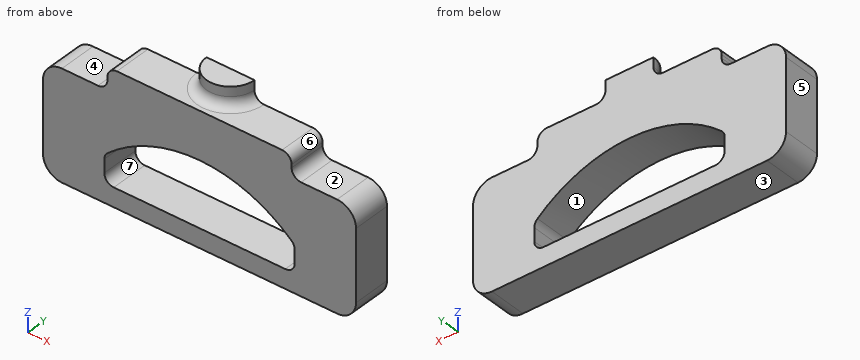
```python
from build123d import *

# Parameters (mm, degrees)
EXTRUDE1_DEPTH = 12.7
EXTRUDE2_DEPTH = 6.35
FILLET1_R      = 3.175


with BuildPart() as part:
    # Sketch1 → Extrude1 (new body)
    with BuildSketch(Plane(origin=(0, 0, 0), x_dir=(1, 0, 0), z_dir=(0, 1, 0))):
        with BuildLine():
            Line((0, 30.076477833), (0, 6.35))
            ThreePointArc((0, 6.35), (1.859871939, 1.859871939), (6.35, 0))
            Line((6.35, 0), (18.40185504, 0))
            ThreePointArc((18.40185504, 0), (20.64691907, -0.92993597), (21.57685504, -3.175))
            Line((21.57685504, -3.175), (21.57685504, -4.269827586))
            ThreePointArc((21.57685504, -4.269827586), (22.506791009, -6.514891616), (24.75185504, -7.444827586))
            Line((24.75185504, -7.444827586), (80.087569325, -7.444827586))
            ThreePointArc((80.087569325, -7.444827586), (82.332633356, -6.514891616), (83.262569325, -4.269827586))
            Line((83.262569325, -4.269827586), (83.262569325, -3.175))
            ThreePointArc((83.262569325, -3.175), (84.192505295, -0.92993597), (86.437569325, 0))
            Line((86.437569325, 0), (98.489424365, 0))
            ThreePointArc((98.489424365, 0), (102.979552425, 1.859871939), (104.839424365, 6.35))
            Line((104.839424365, 6.35), (104.839424365, 30.076477833))
            ThreePointArc((104.839424365, 30.076477833), (102.979552425, 34.566605893), (98.489424365, 36.426477833))
            Line((98.489424365, 36.426477833), (6.35, 36.426477833))
            ThreePointArc((6.35, 36.426477833), (1.859871939, 34.566605893), (0, 30.076477833))
        make_face()
        with BuildLine():
            Line((81.136140344, 30.076477833), (23.703284021, 30.076477833))
            ThreePointArc((23.703284021, 30.076477833), (21.458219991, 29.146541863), (20.528284021, 26.901477833))
            Line((20.528284021, 26.901477833), (20.528284021, 22.476973979))
            ThreePointArc((20.528284021, 22.476973979), (20.807016141, 21.176106051), (21.594272913, 20.103643587))
            ThreePointArc((21.594272913, 20.103643587), (52.419712182, 8.386390066), (83.245151452, 20.103643587))
            ThreePointArc((83.245151452, 20.103643587), (84.032408224, 21.176106051), (84.311140344, 22.476973979))
            Line((84.311140344, 22.476973979), (84.311140344, 26.901477833))
            ThreePointArc((84.311140344, 26.901477833), (83.381204374, 29.146541863), (81.136140344, 30.076477833))
        make_face(mode=Mode.SUBTRACT)
    extrude(amount=-EXTRUDE1_DEPTH)

    # Sketch2 → Extrude2 (add)
    with BuildSketch(Plane.XY.offset(7.444827586)):
        with BuildLine():
            Line((44.389946351, 0), (60.449478013, 0))
            ThreePointArc((60.449478013, 0), (52.419712182, -8.029765831), (44.389946351, 0))
        make_face()
    extrude(amount=EXTRUDE2_DEPTH)

    # Fillet1
    fillet1_edges = [part.edges().sort_by_distance(p)[0] for p in [
        (52.419712182, -8.029765831, 7.444827586),
    ]]
    fillet(fillet1_edges, radius=FILLET1_R)


solid = part.part
```
Here's how the part is built. I have some questions about the finished solid (model axes, mm). Face numbers are marked on the shaded views. A direction names the side the tool comes from. Round coordinates to 2 decimals unless told otherwise and drop trailing zeros. Loops run counter-clockwise (first coordinate to the right, second up) from the corner with the lowest first, then second, coordinate; pieces in that order, holes last.
1. Thinking about a two-plate mould opening in Z: for the marked faces 5, 6 and 7, which applies, released by +Z, released by -Z, zero draft, split by the parting line, or undercut?
Answers:
face 5: zero draft
face 6: released by +Z
face 7: undercut
2. Suppose I cut it at A-A, the plane x = 37. Please give me the cut outline in (y, z), and give its area (3 significant figures).
Answers:
outline: (-12.7, -36.43) - (0, -36.43) - (0, -30.08) - (-12.7, -30.08) - close; (-12.7, -11.02) - (0, -11.02) - (0, 7.44) - (-12.7, 7.44) - close
area: 315 mm2
3. Suppose I cut it at B-B, the plane x = 87.5. Please give me the cut outline in (y, z).
Answers:
outline: (-12.7, -36.43) - (0, -36.43) - (0, 0) - (-12.7, 0) - close
4. If I drill on probe 1 along X at (y, z) = (-10.25, -25); probe 2 along Z at (x, y) = (73, -9); probe 3 along X at (y, z) = (-6.25, -18.5), over which ranges is the centre line in solid material (lowest first)?
Answers:
probe 1: x = 0 to 20.53, 84.31 to 104.84
probe 2: z = -36.43 to -30.08, -13.2 to 7.44
probe 3: x = 0 to 23.5, 81.34 to 104.84
5. Will these pins go through, and if not, where does the flat tip stop? pin 1 (0.5 mm diameter, centred on y = -7, z = 3.5, fed in from -X); pin 2 (5 mm diameter, centred on x = 67, y = -9, fed in from +Z).
Answers:
pin 1: stops at x = 21.58
pin 2: stops at z = 7.44
6. For the marked faces 1, 2, 3 and 4, which set-ups out of +Z, -Z, +X, -X, +Y, -Y let a thin tool reach every point of the face, with its end or its side?
Answers:
face 1: +Y, -Y
face 2: +Z, +X, +Y, -Y
face 3: -Z, +X, -X, +Y, -Y
face 4: +Z, -X, +Y, -Y
